Read the model definition and answer for the solid it produces. Units are mm, in the model's axes. A direction names the side the tool comes from. Coordinates: 2 decimals unless noted, no trailing zeros. Loops run counter-clockwise (first coordinate to the right, second up) from the corner with the lowest first, then second, coordinate; pieces in that order, holes last. Notation, with made-up numbers: (-37, 7) - (-22, 7) arc R16 ccw to (-22, 30) - close; hole circle Ø7 at (31.5, 52). An arc over 180 degrees is marked (long way). Use one line per item in the form item = value. Start each with the question number.
1) Which of the six approach directions +Z, -Z, +X, -X, +Y, -Y give full straight-line access (tool end or side, diameter ignored) to faces 5 (the face through (5, 2, 26)), 6 (the face through (-5, 2, -26)), 7 (the face through (-0.98, 1.48, -24.9)), 8 (the face through (-8.618, 3.014, 20.784))?
2) A cutting plane is placed at D-D (x = -8). Give the vertices of the cut face in (y, z), and give its area (3 significant figures).
3) A cutting plane is placed at B-B (y = 0.6). Give the vertices of the cut face in (x, z), and give its area (3 significant figures).
4) Each of these flat-tipped pins is pushed along its axis until it touches: P1, Ø1.5, axis at y = 3, z = -27, coming from the +X side; P2, Ø2, axis at y = 0.5, z = -16, coming from the +X side; P3, Ø3, axis at x = 1.5, z = -27.5, coming from the -Y side. Where does it stop, or does it pass through?
5) A cutting plane is placed at A-A (z = 0). Give the vertices of the cut face in (x, y), and give its area (3 significant figures).
6) The mould has two halves that part along X. Classify faces 1 (the face through (-5, 2, 27)), 2 (the face through (1.4, 3, -26.6)), 3 (the face through (-4, 0, -20)), 4 (the face through (5, 2, -27)): released by +X, released by -X, zero draft, split by the parting line, or undercut.
7) Consider line 1 (X direction, y = 3.65, z = -28); line 2 (X direction, y = 2.35, z = 8.5); line 3 (Z direction, x = -4, y = 3.75). Determine where each line is inside the solid, lowest interval first.
8) A cutting plane is placed at C-C (x = 0). Give the vertices of the cut face in (y, z).
from build123d import *

# Parameters (mm, degrees)
BOSS_EXTRUDE1_DEPTH = 4
SKETCH2_R           = 20
CUT_EXTRUDE1_DEPTH  = 42.593268686
SKETCH3_R           = 22.5
CUT_EXTRUDE2_DEPTH  = 2
SKETCH4_R           = 1.75
CUT_EXTRUDE3_DEPTH  = 42.593268686
SKETCH5_R           = 3.25
CUT_EXTRUDE4_DEPTH  = 3


with BuildPart() as part:
    # Sketch1 → Boss-Extrude1 (new body)
    with BuildSketch(Plane(origin=(0, 0, 0), x_dir=(1, 0, 0), z_dir=(0, 1, 0))):
        with BuildLine():
            Line((-5, 25), (-5, 28))
            ThreePointArc((-5, 28), (0, 33), (5, 28))
            Line((5, 28), (5, 25))
            ThreePointArc((5, 25), (4.993730366, 24.749686125), (4.974937186, 24.5))
            ThreePointArc((4.974937186, 24.5), (25, 0), (4.974937186, -24.5))
            ThreePointArc((4.974937186, -24.5), (4.993730366, -24.749686125), (5, -25))
            Line((5, -25), (5, -28))
            ThreePointArc((5, -28), (0, -33), (-5, -28))
            Line((-5, -28), (-5, -25))
            ThreePointArc((-5, -25), (-4.993730366, -24.749686125), (-4.974937186, -24.5))
            ThreePointArc((-4.974937186, -24.5), (-25, 0), (-4.974937186, 24.5))
            ThreePointArc((-4.974937186, 24.5), (-4.993730366, 24.749686125), (-5, 25))
        make_face()
    extrude(amount=BOSS_EXTRUDE1_DEPTH)

    # Sketch2 → Cut-Extrude1 (cut, through all)
    with BuildSketch(Plane(origin=(0, 4, 0), x_dir=(1, 0, 0), z_dir=(0, 1, 0))):
        with Locations(Location((0, 0, 0), (0, 0, 270))):
            Circle(SKETCH2_R)
    extrude(amount=-CUT_EXTRUDE1_DEPTH, mode=Mode.SUBTRACT)

    # Sketch3 → Cut-Extrude2 (cut)
    with BuildSketch(Plane(origin=(0, 4, 0), x_dir=(1, 0, 0), z_dir=(0, 1, 0))):
        with Locations(Location((0, 0, 0), (0, 0, 270))):
            Circle(SKETCH3_R)
    extrude(amount=-CUT_EXTRUDE2_DEPTH, mode=Mode.SUBTRACT)

    # Sketch4 → Cut-Extrude3 (cut, through all)
    with BuildSketch(Plane(origin=(0, 4, 0), x_dir=(1, 0, 0), z_dir=(0, 1, 0))):
        with Locations(Location((0, -28, 0), (0, 0, 270))):
            Circle(SKETCH4_R)
        with Locations(Location((0, 28, 0), (0, 0, 90))):
            Circle(SKETCH4_R)
    extrude(amount=-CUT_EXTRUDE3_DEPTH, mode=Mode.SUBTRACT)

    # Sketch5 → Cut-Extrude4 (cut)
    with BuildSketch(Plane.XZ):
        with Locations(Location((0, 28, 0), (0, 0, 270))):
            Circle(SKETCH5_R)
        with Locations(Location((0, -28, 0), (0, 0, 90))):
            Circle(SKETCH5_R)
    extrude(amount=-CUT_EXTRUDE4_DEPTH, mode=Mode.SUBTRACT)


solid = part.part
Found:
q1.face_5 = +Z, +X, +Y, -Y
q1.face_6 = -Z, -X, +Y, -Y
q1.face_7 = -Y
q1.face_8 = +Y
q2.outline = (0, -23.69) - (4, -23.69) - (4, -21.03) - (2, -21.03) - (2, -18.33) - (0, -18.33) - close; (0, 18.33) - (2, 18.33) - (2, 21.03) - (4, 21.03) - (4, 23.69) - (0, 23.69) - close
q2.area = 32.0 mm^2
q3.outline = (-5, -28) arc R5 ccw to (5, -28) - (5, -25) arc R5 ccw to (4.97, -24.5) arc R25 ccw to (4.97, 24.5) arc R5 ccw to (5, 25) - (5, 28) arc R5 ccw to (-5, 28) - (-5, 25) arc R5 ccw to (-4.97, 24.5) arc R25 ccw to (-4.97, -24.5) arc R5 ccw to (-5, -25) - close; hole circle Ø40 at (0, 0); hole circle Ø6.5 at (0, -28); hole circle Ø6.5 at (0, 28)
q3.area = 782 mm^2
q4.P1 = 5
q4.P2 = 20
q4.P3 = 3
q5.outline = (-25, 0) - (-20, 0) - (-20, 2) - (-22.5, 2) - (-22.5, 4) - (-25, 4) - close; (20, 0) - (25, 0) - (25, 4) - (22.5, 4) - (22.5, 2) - (20, 2) - close
q5.area = 30.0 mm^2
q6.face_1 = released by -X
q6.face_2 = undercut
q6.face_3 = zero draft
q6.face_4 = released by +X
q7.line_1 = -5 to -1.75, 1.75 to 5
q7.line_2 = -23.51 to -20.83, 20.83 to 23.51
q7.line_3 = -31 to -22.14, 22.14 to 31
q8.outline = (0, -33) - (4, -33) - (4, -29.75) - (3, -29.75) - (3, -31.25) - (0, -31.25) - close; (0, -24.75) - (3, -24.75) - (3, -26.25) - (4, -26.25) - (4, -22.5) - (2, -22.5) - (2, -20) - (0, -20) - close; (0, 20) - (2, 20) - (2, 22.5) - (4, 22.5) - (4, 26.25) - (3, 26.25) - (3, 24.75) - (0, 24.75) - close; (0, 31.25) - (3, 31.25) - (3, 29.75) - (4, 29.75) - (4, 33) - (0, 33) - close
